```python
from build123d import *

# Parameters (mm, degrees)
SKETCH_1_W          = 46
SKETCH_1_H          = 54
EXTRUDE_1_DEPTH     = 3.6
SKETCH_2_R          = 1.6
SKETCH_2_R_2        = 1.634420344
SKETCH_2_R_3        = 8.5
SKETCH_2_R_4        = 4.1
CUT_EXTRUDE_1_DEPTH = 3.6
SKETCH_4_R          = 4.1
SKETCH_4_R_2        = 2.6
EXTRUDE_2_DEPTH     = 1
SKETCH_5_W          = 10
SKETCH_5_H          = 16
CUT_EXTRUDE_2_DEPTH = 4
CUT_EXTRUDE_3_DEPTH = 10
SKETCH_7_R          = 4.6
SKETCH_7_R_2        = 1.6
EXTRUDE_3_DEPTH     = 3.8
SKETCH_10_R         = 1.6
CUT_EXTRUDE_6_DEPTH = 72.038299529
SKETCH_11_R         = 1.6
CUT_EXTRUDE_7_DEPTH = 72.038299529


with BuildPart() as part:
    # 草图1 → 凸台-拉伸1 (new body)
    with BuildSketch(Plane(origin=(0, 0, 0), x_dir=(1, 0, 0), z_dir=(0, 1, 0))):
        with Locations((23, 27)):
            Rectangle(SKETCH_1_W, SKETCH_1_H)
    extrude(amount=EXTRUDE_1_DEPTH)

    # 草图2 → 切除-拉伸1 (cut)
    with BuildSketch(Plane(origin=(0, 0, 0), x_dir=(-1, 0, 0), z_dir=(0, -1, 0))):
        with Locations(Location((-18.15, 49.3, 0), (0, 0, 90))):
            Circle(SKETCH_2_R)
        with Locations(Location((-18.15, 5.45, 0), (0, 0, 90))):
            Circle(SKETCH_2_R_2)
        with Locations(Location((-18.15, 27.375, 0), (0, 0, 90))):
            Circle(SKETCH_2_R_3)
        with Locations(Location((-33.15, 23.95, 0), (0, 0, 90))):
            Circle(SKETCH_2_R_4)
    extrude(amount=-CUT_EXTRUDE_1_DEPTH, mode=Mode.SUBTRACT)

    # 草图4 → 凸台-拉伸2 (add)
    with BuildSketch(Plane(origin=(0, 0, 0), x_dir=(-1, 0, 0), z_dir=(0, -1, 0))):
        with Locations(Location((-33.15, 23.95, 0), (0, 0, 90))):
            Circle(SKETCH_4_R)
        with Locations(Location((-33.15, 23.95, 0), (0, 0, 90))):
            Circle(SKETCH_4_R_2, mode=Mode.SUBTRACT)
    extrude(amount=-EXTRUDE_2_DEPTH)

    # 草图5 → 切除-拉伸2 (cut)
    with BuildSketch(Plane(origin=(0, 3.6, 0), x_dir=(1, 0, 0), z_dir=(0, 1, 0))):
        with Locations((41, 46)):
            Rectangle(SKETCH_5_W, SKETCH_5_H)
    extrude(amount=-CUT_EXTRUDE_2_DEPTH, mode=Mode.SUBTRACT)

    # 草图6 → 切除-拉伸3 (cut)
    with BuildSketch(Plane(origin=(0, 0, 0), x_dir=(-1, 0, 0), z_dir=(0, -1, 0))):
        with BuildLine():
            ThreePointArc((-22.56285512, 4.064734889), (-18.15, 3.85), (-13.73714488, 4.064734889))
            ThreePointArc((-13.73714488, 4.064734889), (-11.94032174, 5.854871857), (-14.05952591, 7.248477772))
            ThreePointArc((-14.05952591, 7.248477772), (-18.15, 7.05), (-22.24047409, 7.248477772))
            ThreePointArc((-22.24047409, 7.248477772), (-24.35967826, 5.854871857), (-22.56285512, 4.064734889))
        make_face()
        with BuildLine():
            ThreePointArc((-21.330278495, 19.041671333), (-18.15, 18.875), (-14.969721505, 19.041671333))
            ThreePointArc((-14.969721505, 19.041671333), (-7.404777332, 28.383599382), (-16.746705381, 35.948543555))
            ThreePointArc((-16.746705381, 35.948543555), (-18.15, 35.875), (-19.553294619, 35.948543555))
            ThreePointArc((-19.553294619, 35.948543555), (-27.538099682, 28.240960008), (-21.330278495, 19.041671333))
        make_face()
    extrude(amount=-CUT_EXTRUDE_3_DEPTH, mode=Mode.SUBTRACT)

    # 草图7 → 凸台-拉伸3 (add)
    # profile 1 of 2: a face of its own
    with BuildSketch(Plane(origin=(0, 3.6, 0), x_dir=(1, 0, 0), z_dir=(0, 1, 0))):
        with Locations(Location((18.15, 49.3, 0), (0, 0, 90))):
            Circle(SKETCH_7_R)
        with Locations(Location((18.15, 49.3, 0), (0, 0, 90))):
            Circle(SKETCH_7_R_2, mode=Mode.SUBTRACT)
    # profile 2 of 2: a face of its own
    with BuildSketch(Plane(origin=(0, 3.6, 0), x_dir=(1, 0, 0), z_dir=(0, 1, 0))):
        with BuildLine():
            ThreePointArc((18.683380864, 10.053624309), (20.204186283, 10.103790761), (21.721904392, 10.21286658))
            ThreePointArc((21.721904392, 10.21286658), (27.345628596, 6.144963348), (22.624665084, 1.05707438))
            ThreePointArc((22.624665084, 1.05707438), (20.68567708, 0.916399041), (18.742606478, 0.853624309))
            ThreePointArc((18.742606478, 0.853624309), (18.15, 0.815579656), (17.557393522, 0.853624309))
            ThreePointArc((17.557393522, 0.853624309), (15.61432292, 0.916399041), (13.675334916, 1.05707438))
            ThreePointArc((13.675334916, 1.05707438), (8.954371404, 6.144963348), (14.578095608, 10.21286658))
            ThreePointArc((14.578095608, 10.21286658), (16.095813717, 10.103790761), (17.616619136, 10.053624309))
            ThreePointArc((17.616619136, 10.053624309), (18.15, 10.084420344), (18.683380864, 10.053624309))
        make_face()
        with BuildLine():
            ThreePointArc((18.477514951, 7.05126944), (20.361194151, 7.107902157), (22.24047409, 7.248477772))
            ThreePointArc((22.24047409, 7.248477772), (24.35967826, 5.854871857), (22.56285512, 4.064734889))
            ThreePointArc((22.56285512, 4.064734889), (20.528669211, 3.912287645), (18.489691709, 3.85126944))
            ThreePointArc((18.489691709, 3.85126944), (18.15, 3.815579656), (17.810308291, 3.85126944))
            ThreePointArc((17.810308291, 3.85126944), (15.771330789, 3.912287645), (13.73714488, 4.064734889))
            ThreePointArc((13.73714488, 4.064734889), (11.94032174, 5.854871857), (14.05952591, 7.248477772))
            ThreePointArc((14.05952591, 7.248477772), (15.938805849, 7.107902157), (17.822485049, 7.05126944))
            ThreePointArc((17.822485049, 7.05126944), (18.15, 7.084420344), (18.477514951, 7.05126944))
        make_face(mode=Mode.SUBTRACT)
    extrude(amount=EXTRUDE_3_DEPTH)

    # 草图10 → 切除-拉伸6 (cut, through all)
    with BuildSketch(Plane(origin=(0, 3.6, 0), x_dir=(1, 0, 0), z_dir=(0, 1, 0))):
        with Locations(Location((42, 8.95, 0), (0, 0, 270))):
            Circle(SKETCH_10_R)
    extrude(amount=-CUT_EXTRUDE_6_DEPTH, mode=Mode.SUBTRACT)

    # 草图11 → 切除-拉伸7 (cut, through all)
    with BuildSketch(Plane(origin=(0, 3.6, 0), x_dir=(1, 0, 0), z_dir=(0, 1, 0))):
        with Locations(Location((31.95, 48, 0), (0, 0, 270))):
            Circle(SKETCH_11_R)
    extrude(amount=-CUT_EXTRUDE_7_DEPTH, mode=Mode.SUBTRACT)


solid = part.part
```
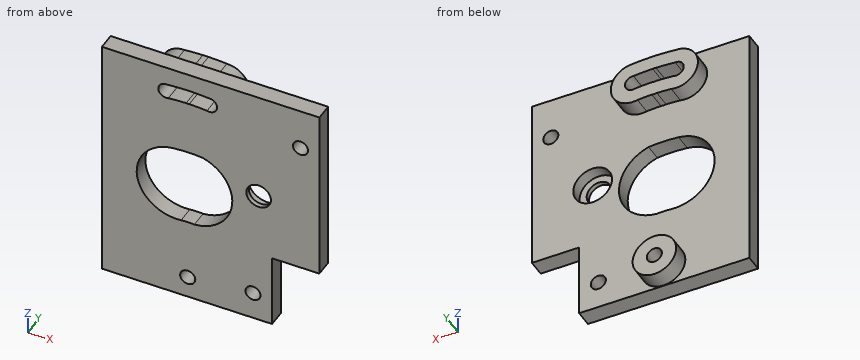
Input: part model. Units: mm. Frame: model coordinates. Give positions to 0.01 mm unless a question says otherwise; leave off trailing zeros. Write each loop counter-clockwise with the first axis right and the second up, starting at its lowest first coordinate (ties: lowest second). Pieces come first, ordered by that corner, then holes. Notation, with made-up numbers: (33.25, 55) - (89.25, 55) arc R22 cw to (89.25, 93) - close; hole circle Ø1 at (77.5, 58). An arc over 180 degrees is marked (long way). Write item = value, one per line. Start each with the question number.
1. Ray query, L1, parallel to X at y = 5.45, z = -49.3; L2, parallel to X at y = 0.8, z = -23.95; L3, parallel to Z at x = 15, y = 5.25. Return the intervals inside material, ascending.
2. Section query A-A, the plane y = 4.25. Output: boundary loops of the cut face in (x, z).
3. Section query B-B, the plane x = 42. Output: boundary loops of the cut face in (y, z), then the cut area to 3 significant figures.
4. Section query C-C, the plane z = -35. Output: boundary loops of the cut face in (x, y).
5. Section query D-D, the plane x = 31.95. Output: boundary loops of the cut face in (y, z).
6. First-contact query: pin 1 Ø1.8 at (x, y) = (39, 2) entering from -Z; pin 2 Ø4 at (x, z) = (28.5, -32.5) entering from +Y; pin 3 Ø1.1 at (y, z) = (2, -44.5) entering from +X. Flat tips, straight axial feed; report the tip coordinate or a pass-through.
Check sheet entries:
q1.L1 = 13.55 to 16.55, 19.75 to 22.75
q1.L2 = 0 to 8.13, 26.89 to 30.55, 35.75 to 46
q1.L3 = -52.65 to -45.95, -10.18 to -7.17, -3.96 to -0.95
q2.outline = circle Ø9.2 at (18.15, -49.3); (13.68, -1.06) arc R4.63 ccw (long way) to (14.58, -10.21) arc R39.25 cw to (17.62, -10.05) arc R4.63 ccw to (18.68, -10.05) arc R39.25 cw to (21.72, -10.21) arc R4.63 ccw (long way) to (22.62, -1.06) arc R48.45 ccw to (18.74, -0.85) arc R4.63 ccw to (17.56, -0.85) arc R48.45 ccw to start; hole (13.74, -4.06) arc R1.63 ccw (long way) to (14.06, -7.25) arc R42.25 cw to (17.82, -7.05) arc R1.63 ccw to (18.48, -7.05) arc R42.25 cw to (22.24, -7.25) arc R1.63 ccw (long way) to (22.56, -4.06) arc R45.45 ccw to (18.49, -3.85) arc R1.63 ccw to (17.81, -3.85) arc R45.45 ccw to start; hole circle Ø3.2 at (18.15, -49.3)
q3.outline = (0, -38) - (3.6, -38) - (3.6, -10.55) - (0, -10.55) - close; (0, -7.35) - (3.6, -7.35) - (3.6, 0) - (0, 0) - close
q3.area = 125 mm2
q4.outline = (0, 0) - (11.87, 0) - (11.87, 3.6) - (0, 3.6) - close; (22.93, 0) - (46, 0) - (46, 3.6) - (22.93, 3.6) - close
q5.outline = (0, -54) - (3.6, -54) - (3.6, -49.6) - (0, -49.6) - close; (0, -46.4) - (3.6, -46.4) - (3.6, -27.87) - (1, -27.87) - (1, -26.26) - (0, -26.26) - close; (0, -21.64) - (1, -21.64) - (1, -20.03) - (3.6, -20.03) - (3.6, 0) - (0, 0) - close
q6.pin_1 = -38
q6.pin_2 = 3.6
q6.pin_3 = 36
